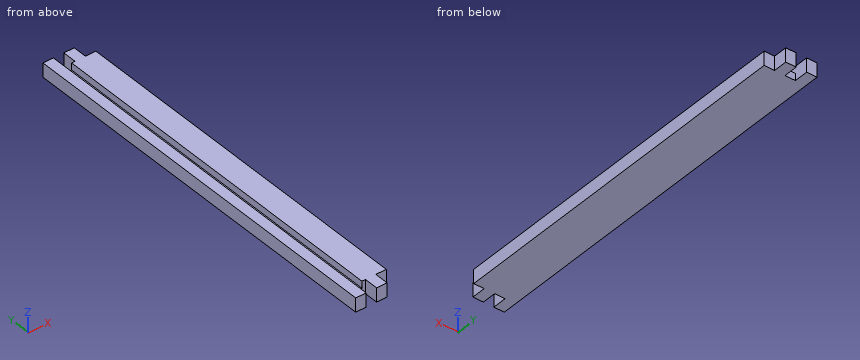
from build123d import *

# Parameters (mm, degrees)
F0_W     = 38.1
F0_H     = 12.7
F1_DEPTH = 355.6
F2_W     = 6.35
F2_H     = 6.35
F3_DEPTH = 355.601
F4_W     = 9.525
F4_H     = 12.7
F5_DEPTH = 12.701


with BuildPart() as f1:
    # F0 (on Front) → F1 (new body)
    with BuildSketch(Plane.XZ):
        with Locations((19.05, 6.35)):
            Rectangle(F0_W, F0_H)
    extrude(amount=F1_DEPTH)

    # F2 (on face) → F3 (cut, through all)
    with BuildSketch(Plane.XZ.offset(355.6)):
        with Locations((12.7, 9.525)):
            Rectangle(F2_W, F2_H)
    extrude(amount=-F3_DEPTH, mode=Mode.SUBTRACT)

    # F4 (on face) → F5 (cut, through all)
    with BuildSketch(Plane(origin=(0, 0, 0), x_dir=(1, 0, 0), z_dir=(0, 0, -1))):
        with Locations((33.3375, 349.25)):
            Rectangle(F4_W, F4_H)
        with Locations((14.2875, 349.25)):
            Rectangle(F4_W, F4_H)
        with Locations((33.3375, 6.35)):
            Rectangle(F4_W, F4_H)
        with Locations((14.2875, 6.35)):
            Rectangle(F4_W, F4_H)
    extrude(amount=-F5_DEPTH, mode=Mode.SUBTRACT)


solid = f1.part
The listing builds one solid part. Answer for the finished solid, in the listing's coordinates (mm). Give positions to 0.01 mm unless a question says otherwise; leave off trailing zeros. Loops run counter-clockwise (first coordinate to the right, second up) from the corner with the lowest first, then second, coordinate; pieces in that order, holes last. Notation, with made-up numbers: (18, -23.75) - (36, -23.75) arc R16 cw to (36, 3.25) - close; hole circle Ø8 at (3, -18). An arc over 180 degrees is marked (long way). Use one line per item in the form item = value.
1. Given pin 1 Ø7.5 at (x, z) = (33.5, 3.5) entering from -Y; pin 2 Ø7.5 at (x, z) = (14, 7) entering from +Y; pin 3 Ø1.9 at (x, y) = (11.5, -201) entering from +Z, each flat-ended and moving along its own axis, determine where each tip first touches the part or whether it passes through.
Calculated:
pin_1 = -342.9
pin_2 = -12.7
pin_3 = 6.35
2. Section C-C on x = 32.5 is taken. Give the vertices of the cut face in (y, z), then the cut area to 3 significant figures.
Calculated:
outline = (-342.9, 0) - (-12.7, 0) - (-12.7, 12.7) - (-342.9, 12.7) - close
area = 4,190 mm^2
3. Section D-D on x = 13 is taken. Give the vertices of the cut face in (y, z).
Calculated:
outline = (-342.9, 0) - (-12.7, 0) - (-12.7, 6.35) - (-342.9, 6.35) - close
4. Section B-B on y = -170.5 is taken. Give the vertices of the cut face in (x, z) (3 decimals).
Calculated:
outline = (0, 0) - (38.1, 0) - (38.1, 12.7) - (15.875, 12.7) - (15.875, 6.35) - (9.525, 6.35) - (9.525, 12.7) - (0, 12.7) - close
5. Section A-A on z = 10 is taken. Give the vertices of the cut face in (x, y) (3 decimals), then the cut area to 3 significant figures.
Calculated:
outline = (0, -355.6) - (9.525, -355.6) - (9.525, 0) - (0, 0) - close; (15.875, -342.9) - (19.05, -342.9) - (19.05, -355.6) - (28.575, -355.6) - (28.575, -342.9) - (38.1, -342.9) - (38.1, -12.7) - (28.575, -12.7) - (28.575, 0) - (19.05, 0) - (19.05, -12.7) - (15.875, -12.7) - close
area = 11,000 mm^2
6. Find the intervals of material crossed by line 1 along X through (y, z) = (-38, 8.75) (3 decimals); line 2 along Y through (x, z) = (29.5, 10.75), in increasing order. Write a range as [from, to].
Calculated:
line_1 = [0, 9.525], [15.875, 38.1]
line_2 = [-342.9, -12.7]
